from build123d import *

# Parameters (mm, degrees)
SKETCH2_R           = 10.8077
BOSS_EXTRUDE1_DEPTH = 5.1308


with BuildPart() as part:
    # Sketch2 → Boss-Extrude1 (new body)
    with BuildSketch(Plane(origin=(0, 0, 0), x_dir=(1, 0, 0), z_dir=(0, 1, 0))):
        with BuildLine():
            Line((-17.306656678, 35.509756676), (-10.733030501, 22.022006247))
            ThreePointArc((-10.733030501, 22.022006247), (-13.61052624, 20.369592003), (-16.238327885, 18.34348414))
            Line((-16.238327885, 18.34348414), (-26.183766617, 29.578261448))
            ThreePointArc((-26.183766617, 29.578261448), (-27.932625947, 27.932625947), (-29.578261448, 26.183766617))
            Line((-29.578261448, 26.183766617), (-18.34348414, 16.238327885))
            ThreePointArc((-18.34348414, 16.238327885), (-20.369592003, 13.61052624), (-22.022006247, 10.733030501))
            Line((-22.022006247, 10.733030501), (-35.509756676, 17.306656678))
            ThreePointArc((-35.509756676, 17.306656678), (-36.495734573, 15.117028229), (-37.34684404, 12.871535447))
            Line((-37.34684404, 12.871535447), (-23.161308603, 7.982511303))
            ThreePointArc((-23.161308603, 7.982511303), (-24.027572035, 4.779381236), (-24.453033788, 1.488570263))
            Line((-24.453033788, 1.488570263), (-39.429708177, 2.400270314))
            ThreePointArc((-39.429708177, 2.400270314), (-39.502698446, 0), (-39.429708177, -2.400270314))
            Line((-39.429708177, -2.400270314), (-24.453033788, -1.488570263))
            ThreePointArc((-24.453033788, -1.488570263), (-24.027572035, -4.779381236), (-23.161308603, -7.982511303))
            Line((-23.161308603, -7.982511303), (-37.34684404, -12.871535447))
            ThreePointArc((-37.34684404, -12.871535447), (-36.495734573, -15.117028229), (-35.509756676, -17.306656678))
            Line((-35.509756676, -17.306656678), (-22.022006247, -10.733030501))
            ThreePointArc((-22.022006247, -10.733030501), (-20.369592003, -13.61052624), (-18.34348414, -16.238327885))
            Line((-18.34348414, -16.238327885), (-29.578261448, -26.183766617))
            ThreePointArc((-29.578261448, -26.183766617), (-27.932625947, -27.932625947), (-26.183766617, -29.578261448))
            Line((-26.183766617, -29.578261448), (-16.238327885, -18.34348414))
            ThreePointArc((-16.238327885, -18.34348414), (-13.61052624, -20.369592003), (-10.733030501, -22.022006247))
            Line((-10.733030501, -22.022006247), (-17.306656678, -35.509756676))
            ThreePointArc((-17.306656678, -35.509756676), (-15.117028229, -36.495734573), (-12.871535447, -37.34684404))
            Line((-12.871535447, -37.34684404), (-7.982511303, -23.161308603))
            ThreePointArc((-7.982511303, -23.161308603), (-4.779381236, -24.027572035), (-1.488570263, -24.453033788))
            Line((-1.488570263, -24.453033788), (-2.400270314, -39.429708177))
            ThreePointArc((-2.400270314, -39.429708177), (0, -39.502698446), (2.400270314, -39.429708177))
            Line((2.400270314, -39.429708177), (1.488570263, -24.453033788))
            ThreePointArc((1.488570263, -24.453033788), (4.779381236, -24.027572035), (7.982511303, -23.161308603))
            Line((7.982511303, -23.161308603), (12.871535447, -37.34684404))
            ThreePointArc((12.871535447, -37.34684404), (15.117028229, -36.495734573), (17.306656678, -35.509756676))
            Line((17.306656678, -35.509756676), (10.733030501, -22.022006247))
            ThreePointArc((10.733030501, -22.022006247), (13.61052624, -20.369592003), (16.238327885, -18.34348414))
            Line((16.238327885, -18.34348414), (26.183766617, -29.578261448))
            ThreePointArc((26.183766617, -29.578261448), (27.932625947, -27.932625947), (29.578261448, -26.183766617))
            Line((29.578261448, -26.183766617), (18.34348414, -16.238327885))
            ThreePointArc((18.34348414, -16.238327885), (20.369592003, -13.61052624), (22.022006247, -10.733030501))
            Line((22.022006247, -10.733030501), (35.509756676, -17.306656678))
            ThreePointArc((35.509756676, -17.306656678), (36.495734573, -15.117028229), (37.34684404, -12.871535447))
            Line((37.34684404, -12.871535447), (23.161308603, -7.982511303))
            ThreePointArc((23.161308603, -7.982511303), (24.027572035, -4.779381236), (24.453033788, -1.488570263))
            Line((24.453033788, -1.488570263), (39.429708177, -2.400270314))
            ThreePointArc((39.429708177, -2.400270314), (39.502698446, 0), (39.429708177, 2.400270314))
            Line((39.429708177, 2.400270314), (24.453033788, 1.488570263))
            ThreePointArc((24.453033788, 1.488570263), (24.027572035, 4.779381236), (23.161308603, 7.982511303))
            Line((23.161308603, 7.982511303), (37.34684404, 12.871535447))
            ThreePointArc((37.34684404, 12.871535447), (36.495734573, 15.117028229), (35.509756676, 17.306656678))
            Line((35.509756676, 17.306656678), (22.022006247, 10.733030501))
            ThreePointArc((22.022006247, 10.733030501), (20.369592003, 13.61052624), (18.34348414, 16.238327885))
            Line((18.34348414, 16.238327885), (29.578261448, 26.183766617))
            ThreePointArc((29.578261448, 26.183766617), (27.932625947, 27.932625947), (26.183766617, 29.578261448))
            Line((26.183766617, 29.578261448), (16.238327885, 18.34348414))
            ThreePointArc((16.238327885, 18.34348414), (13.61052624, 20.369592003), (10.733030501, 22.022006247))
            Line((10.733030501, 22.022006247), (17.306656678, 35.509756676))
            ThreePointArc((17.306656678, 35.509756676), (15.117028229, 36.495734573), (12.871535447, 37.34684404))
            Line((12.871535447, 37.34684404), (7.982511303, 23.161308603))
            ThreePointArc((7.982511303, 23.161308603), (4.779381236, 24.027572035), (1.488570263, 24.453033788))
            Line((1.488570263, 24.453033788), (2.400270314, 39.429708177))
            ThreePointArc((2.400270314, 39.429708177), (0, 39.502698446), (-2.400270314, 39.429708177))
            Line((-2.400270314, 39.429708177), (-1.488570263, 24.453033788))
            ThreePointArc((-1.488570263, 24.453033788), (-4.779381236, 24.027572035), (-7.982511303, 23.161308603))
            Line((-7.982511303, 23.161308603), (-12.871535447, 37.34684404))
            ThreePointArc((-12.871535447, 37.34684404), (-15.117028229, 36.495734573), (-17.306656678, 35.509756676))
        make_face()
        with Locations(Location((0, 0, 0), (0, 0, 270))):
            Circle(SKETCH2_R, mode=Mode.SUBTRACT)
    extrude(amount=BOSS_EXTRUDE1_DEPTH)


solid = part.part
Build history of the part. All positions in model axes, mm. A direction names the side the tool comes from. Coordinates: 2 decimals unless noted, no trailing zeros. Write each loop counter-clockwise with the first axis right and the second up, starting at its lowest first coordinate (ties: lowest second). Pieces come first, ordered by that corner, then holes.
(1) Cut at D-D on z = -32. List the corners of the cut face in (x, y).
(2) Cut at A-A on z = 0. List the corners of the cut face in (x, y).
(3) 3-axis set-ups, long thin cutter, end or side, ignore diameter. For faces 4 (the flat face through (-10.46, 2.53, 30.35)), 5 (the cylindrical face through (-36.509, 2.529, 15.086)), 6 (the flat face through (13.974, 2.529, -28.671)): which of +Z, -Z, +X, -X, +Y, -Y reach the whole face in a straight line?
(4) Pin check, flat tips, straight feed: pin 1 Ø3 at (x, z) = (27, -23.5) entering from -Y; pin 2 Ø1.5 at (x, z) = (13.5, 24.5) entering from +Y; pin 3 Ø3 at (x, y) = (23.5, 4) entering from +Z; pin 4 Ø1.5 at (x, y) = (-29.5, 1) entering from -Z. Stop position of each tip, or through.
(5) Cut at C-C on x = -32.5. List the corners of the cut face in (y, z), and give its area (3 significant figures).
(6) Mould opens along X. For faces 1 (the cylindrical face through (-36.48, 2.53, -15.15)), 2 (the flat face through (30.35, 2.53, 10.46)), 3 (the flat face through (-1.94, 2.53, 31.84)) say: pulls with the +X half, pulls with the -X half, needs draft (parallel to the pull), parting line crosses it, or undercut.
(7) Cut at B-B on x = 0. List the corners of the cut face in (y, z), and give its area (3 significant figures).
(8) Drill centre lines: line 1 (Z direction, x = 16.5, y = 3.75); line 2 (X direction, y = 3.1, z = 0); line 3 (X direction, y = 2.8, z = -35). Where is each one in solid material? Low to high.
Working result:
1. outline: (-15.6, 0) - (-11.03, 0) - (-11.03, 5.13) - (-15.6, 5.13) - close; (-1.95, 0) - (1.95, 0) - (1.95, 5.13) - (-1.95, 5.13) - close; (11.03, 0) - (15.6, 0) - (15.6, 5.13) - (11.03, 5.13) - close
2. outline: (-39.5, 0) - (-10.81, 0) - (-10.81, 5.13) - (-39.5, 5.13) - close; (10.81, 0) - (39.5, 0) - (39.5, 5.13) - (10.81, 5.13) - close
3. face 4: +Z, +Y, -Y
3. face 5: +Z, -X, +Y, -Y
3. face 6: +Y, -Y
4. pin 1: stops at y = 0
4. pin 2: passes through
4. pin 3: stops at z = 28.24
4. pin 4: stops at z = -27.09
5. outline: (0, -15.84) - (5.13, -15.84) - (5.13, -11.2) - (0, -11.2) - close; (0, -1.98) - (5.13, -1.98) - (5.13, 1.98) - (0, 1.98) - close; (0, 11.2) - (5.13, 11.2) - (5.13, 15.84) - (0, 15.84) - close
5. area: 67.9 mm2
6. face 1: pulls with the -X half
6. face 2: pulls with the +X half
6. face 3: undercut
7. outline: (0, -39.5) - (5.13, -39.5) - (5.13, -10.81) - (0, -10.81) - close; (0, 10.81) - (5.13, 10.81) - (5.13, 39.5) - (0, 39.5) - close
7. area: 294 mm2
8. line 1: z = -35.89 to -33.85, -18.64 to 18.64, 33.85 to 35.89
8. line 2: x = -39.5 to -10.81, 10.81 to 39.5
8. line 3: x = -17.06 to -12.06, -2.13 to 2.13, 12.06 to 17.06
